```python
from build123d import *

# Parameters (mm, degrees)
F1_DEPTH = 3


with BuildPart() as f1:
    # F0 (on Top) → F1 (new body)
    with BuildSketch(Plane.XY):
        with BuildLine():
            Line((17.2046505341, 14.5), (-17.2046505341, 14.5))
            ThreePointArc((-17.2046505341, 14.5), (-18.4252352643, 12.9135860804), (-19.5, 11.2249721603))
            Line((-19.5, 11.2249721603), (-19.5, 1.25))
            ThreePointArc((-19.5, 1.25), (-18.6161165235, 0.8838834765), (-18.25, 0))
            ThreePointArc((-18.25, 0), (-18.6161165235, -0.8838834765), (-19.5, -1.25))
            Line((-19.5, -1.25), (-19.5, -11.2249721603))
            ThreePointArc((-19.5, -11.2249721603), (-14.0403252344, -17.5817879441), (-6.6332495807, -21.5))
            Line((-6.6332495807, -21.5), (6.6332495807, -21.5))
            ThreePointArc((6.6332495807, -21.5), (14.0403252344, -17.5817879441), (19.5, -11.2249721603))
            Line((19.5, -11.2249721603), (19.5, -1.25))
            ThreePointArc((19.5, -1.25), (18.25, 0), (19.5, 1.25))
            Line((19.5, 1.25), (19.5, 11.2249721603))
            ThreePointArc((19.5, 11.2249721603), (18.4252352643, 12.9135860804), (17.2046505341, 14.5))
        make_face()
        with BuildLine():
            Line((14.1421356237, 17.5), (-14.1421356237, 17.5))
            ThreePointArc((-14.1421356237, 17.5), (-15.7450071644, 16.0731064015), (-17.2046505341, 14.5))
            Line((-17.2046505341, 14.5), (17.2046505341, 14.5))
            ThreePointArc((17.2046505341, 14.5), (15.7450071644, 16.0731064015), (14.1421356237, 17.5))
        make_face()
        with BuildLine():
            Line((-19.5, 1.25), (-19.5, 11.2249721603))
            ThreePointArc((-19.5, 11.2249721603), (-22.5, 0), (-19.5, -11.2249721603))
            Line((-19.5, -11.2249721603), (-19.5, -1.25))
            ThreePointArc((-19.5, -1.25), (-20.75, 0), (-19.5, 1.25))
        make_face()
        with BuildLine():
            ThreePointArc((19.5, -11.2249721603), (22.5, 0), (19.5, 11.2249721603))
            Line((19.5, 11.2249721603), (19.5, 1.25))
            ThreePointArc((19.5, 1.25), (20.3838834765, 0.8838834765), (20.75, 0))
            ThreePointArc((20.75, 0), (20.3838834765, -0.8838834765), (19.5, -1.25))
            Line((19.5, -1.25), (19.5, -11.2249721603))
        make_face()
    extrude(amount=F1_DEPTH)


solid = f1.part
```
Input: part model. Units: mm. Frame: model coordinates. Round coordinates to 2 decimals unless told otherwise and drop trailing zeros. Loops run counter-clockwise (first coordinate to the right, second up) from the corner with the lowest first, then second, coordinate; pieces in that order, holes last. Notation, with made-up numbers: M 78,50 L 123,50 A38 ccw 123,89 Z; hole C -39.75,76.5 d5. An arc over 180 degrees is marked long. Answer in a Markdown table with one row per item. Add a question column.
1. Section B-B (y = 13.5). Output: boundary loops of the cut face in (x, z).
2. Section C-C (x = 15.5). Output: boundary loops of the cut face in (y, z), and give its area (3 significant figures).
3. Ray query, probe 1 along X at (y, z) = (0.5, 2.3); probe 2 along X at (y, z) = (-14.5, 2.25); probe 3 along Y at (x, z) = (-19.5, 1.1). Return the intervals inside material, ascending.
4. Section A-A (z = 0.8). Output: boundary loops of the cut face in (x, y).
Values follow:
| question | item | result |
|---|---|---|
| 1 | outline | M -18,0 L 18,0 L 18,3 L -18,3 Z |
| 2 | outline | M -16.31,0 L 16.31,0 L 16.31,3 L -16.31,3 Z |
| 2 | area | 97.9 mm^2 |
| 3 | probe 1 | -22.49 to -20.65, -18.35 to 18.35, 20.65 to 22.49 |
| 3 | probe 2 | -17.2 to 17.2 |
| 3 | probe 3 | -11.22 to -1.25, 1.25 to 11.22 |
| 4 | outline | M -14.14,17.5 A22.5 ccw -6.63,-21.5 L 6.63,-21.5 A22.5 ccw 14.14,17.5 Z; hole C -19.5,0 d2.5; hole C 19.5,0 d2.5 |
